Study the drawing (mm; zero at the part's minimum x, y, z) and answer. Give positions to 0.01 mm unless a question says otherwise; leave off trailing zeros. Order: outer loops, then holes, each group sorted by start corner. A loop starts at its lowest first (then second) coordinate and runs counter-clockwise, first axis right, second up. Notation, with made-up numbers: (65.5, -36) -> (72.5, -36) arc R16 ccw to (72.5, -24) -> close; hole circle Ø3 at (83, -34.75). An arc over 180 degrees is marked (long way). Use a Markdown table: item, result. Add a question column.
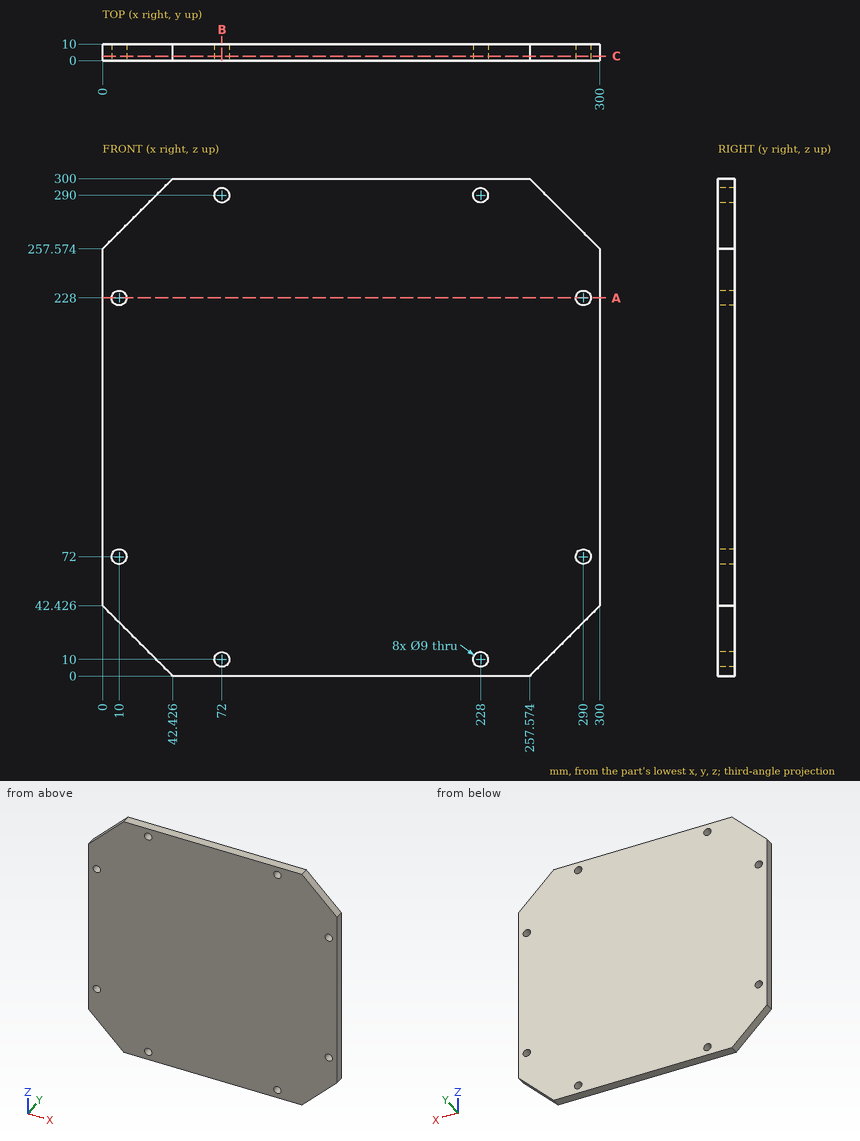
1) The part is cut by section C-C, the plane y = 2.75. State how many separate pieces and enclosed holes the cut face has, then the cut area to 3 significant figures.
2) The part is cut by section A-A, the plane z = 228. Determine the outline of the cut face in (x, y), then the cut area to 3 significant figures.
3) The part is cut by section B-B, the plane x = 72. Determine the outline of the cut face in (y, z), then the cut area to 3 significant figures.
4) Straight lines are drawn through the part: line 1 (X direction, y = 6.5, z = 290) (1 decimal); line 2 (X direction, y = 8.5, z = 227). For each, find the intervals that lie inside material, in ascending order.
A:
| question | item | result |
|---|---|---|
| 1 | separate pieces | 1 |
| 1 | enclosed holes | 8 |
| 1 | area | 85,900 mm^2 |
| 2 | outline | (0, 0) -> (5.5, 0) -> (5.5, 10) -> (0, 10) -> close; (14.5, 0) -> (285.5, 0) -> (285.5, 10) -> (14.5, 10) -> close; (294.5, 0) -> (300, 0) -> (300, 10) -> (294.5, 10) -> close |
| 2 | area | 2,820 mm^2 |
| 3 | outline | (0, 0) -> (10, 0) -> (10, 5.5) -> (0, 5.5) -> close; (0, 14.5) -> (10, 14.5) -> (10, 285.5) -> (0, 285.5) -> close; (0, 294.5) -> (10, 294.5) -> (10, 300) -> (0, 300) -> close |
| 3 | area | 2,820 mm^2 |
| 4 | line 1 | 32.4 to 67.5, 76.5 to 223.5, 232.5 to 267.6 |
| 4 | line 2 | 0 to 5.61, 14.39 to 285.61, 294.39 to 300 |
